Part model, mm, in its own coordinate system. Face numbers are marked on the shaded views. A direction names the side the tool comes from. Round coordinates to 2 decimals unless told otherwise and drop trailing zeros. Loops run counter-clockwise (first coordinate to the right, second up) from the corner with the lowest first, then second, coordinate; pieces in that order, holes last.
1) Band-saw the part on A-A, the plane y = 36. Write the cut outline in (x, z).
2) Band-saw the part on D-D, the plane z = -36. Write the cut outline in (x, y).
3) Drop a flat-ended pin along its axis: P1, Ø5, axis at x = -22, z = -36.5, coming from the +Y side. Give the stop position or say it passes through.
4) Band-saw the part on B-B, the plane z = 0.5. Write the cut outline in (x, y).
5) 3-axis set-ups, long thin cutter, end or side, ignore diameter. For the marked faces 1 and 2: which of +Z, -Z, +X, -X, +Y, -Y reach the whole face in a straight line?
6) Band-saw the part on C-C, the plane x = 7. Write the cut outline in (y, z).
7) Mould opens along Z. For the marked faces 3, 4, 5 and 6 say: +Z half, -Z half, draft (parallel to the pull), parting line (faces both ways), or undercut.
8) Probe line 1 (Z direction, x = 26, y = 20); line 2 (Z direction, x = -4, y = 2). List the from-to ranges inside material, lowest first.
from build123d import *

# Parameters (mm, degrees)
SKETCH1_W               = 100
SKETCH1_H               = 100
BOSS_EXTRUDE1_DEPTH     = 4
SKETCH2_W               = 100
SKETCH2_H               = 100
SKETCH2_W_2             = 92
SKETCH2_H_2             = 92
BOSS_EXTRUDE2_DEPTH     = 35
SKETCH3_W               = 4
SKETCH3_H               = 4
CUT_EXTRUDE1_DEPTH      = 4
BOSS_EXTRUDE3_DEPTH     = 2.5
SKETCH5_W               = 5.75
SKETCH5_H               = 4
CUT_EXTRUDE2_DEPTH      = 4
CUT_EXTRUDE3_DEPTH      = 79.89866919
CUT_EXTRUDE3_DEPTH_BACK = 79.89866919
SKETCH7_W               = 9.25
SKETCH7_H               = 7.5
SKETCH8_W               = 6.199178059
SKETCH8_H               = 6.70376232
SKETCH8_W_2             = 7.56876391
SKETCH8_H_2             = 7.20834658
CUT_EXTRUDE5_DEPTH      = 10
SKETCH9_W               = 12
SKETCH9_H               = 8
CUT_EXTRUDE6_DEPTH      = 10
SKETCH10_W              = 4
SKETCH10_H              = 4
BOSS_EXTRUDE4_DEPTH     = 4
SKETCH11_OUTSIDE_W      = 131.34
SKETCH11_OUTSIDE_H      = 131.34
SKETCH11_OUTSIDE_W_2    = 96
SKETCH11_OUTSIDE_H_2    = 96
CUT_EXTRUDE7_DEPTH      = 81.752708933
SKETCH12_W              = 2
SKETCH12_H              = 8
BOSS_EXTRUDE5_DEPTH     = 2


with BuildPart() as part:
    # Sketch1 → Boss-Extrude1 (new body)
    with BuildSketch(Plane(origin=(0, 0, 0), x_dir=(1, 0, 0), z_dir=(0, 1, 0))):
        Rectangle(SKETCH1_W, SKETCH1_H)
    extrude(amount=BOSS_EXTRUDE1_DEPTH)

    # Sketch2 → Boss-Extrude2 (add)
    with BuildSketch(Plane(origin=(0, 4, 0), x_dir=(1, 0, 0), z_dir=(0, 1, 0))):
        Rectangle(SKETCH2_W, SKETCH2_H)
        Rectangle(SKETCH2_W_2, SKETCH2_H_2, mode=Mode.SUBTRACT)
    extrude(amount=BOSS_EXTRUDE2_DEPTH)

    # Sketch3 → Cut-Extrude1 (cut)
    with BuildSketch(Plane(origin=(0, 0, -50), x_dir=(-1, 0, 0), z_dir=(0, 0, -1))):
        with Locations((0, 37)):
            Rectangle(SKETCH3_W, SKETCH3_H)
    extrude(amount=-CUT_EXTRUDE1_DEPTH, mode=Mode.SUBTRACT)

    # Sketch4 → Boss-Extrude3 (add)
    with BuildSketch(Plane(origin=(0, 4, 0), x_dir=(1, 0, 0), z_dir=(0, 1, 0))):
        Polygon((-1.75, -0.5), (0.75, -0.5), (0.75, 2), (-4.25, 2), (-4.25, -3), (-1.75, -3), align=None)
        Polygon((7.25, -0.5), (9.75, -0.5), (9.75, -3), (12.25, -3), (12.25, 2), (7.25, 2), align=None)
        Polygon((12.25, -14.5), (9.75, -14.5), (9.75, -17), (7.25, -17), (7.25, -19.5), (12.25, -19.5), align=None)
        Polygon((-1.75, -17), (-1.75, -14.5), (-4.25, -14.5), (-4.25, -19.5), (0.75, -19.5), (0.75, -17), align=None)
    extrude(amount=BOSS_EXTRUDE3_DEPTH)

    # Sketch5 → Cut-Extrude2 (cut)
    with BuildSketch(Plane(origin=(0, 4, 0), x_dir=(1, 0, 0), z_dir=(0, 1, 0))):
        with Locations((1.125, -15)):
            Rectangle(SKETCH5_W, SKETCH5_H)
    extrude(amount=-CUT_EXTRUDE2_DEPTH, mode=Mode.SUBTRACT)

    # Sketch7 → Cut-Extrude3 (cut, two sides: drawn at the far end of the back side and taken through both)
    with BuildSketch(Plane(origin=(0, 4, 0), x_dir=(1, 0, 0), z_dir=(0, 1, 0)).offset(-CUT_EXTRUDE3_DEPTH_BACK)):
        with Locations((0.375, -15.75)):
            Rectangle(SKETCH7_W, SKETCH7_H)
        with Locations((7.625, -1.75)):
            Rectangle(SKETCH7_W, SKETCH7_H)
    extrude(amount=CUT_EXTRUDE3_DEPTH + CUT_EXTRUDE3_DEPTH_BACK, mode=Mode.SUBTRACT)

    # Sketch8 → Cut-Extrude5 (cut)
    with BuildSketch(Plane(origin=(0, 4, 0), x_dir=(1, 0, 0), z_dir=(0, 1, 0))):
        with Locations((-1.640574957, -0.408162103)):
            Rectangle(SKETCH8_W, SKETCH8_H)
        with Locations((10.072988236, -16.951317505)):
            Rectangle(SKETCH8_W_2, SKETCH8_H_2)
    extrude(amount=CUT_EXTRUDE5_DEPTH, mode=Mode.SUBTRACT)

    # Sketch9 → Cut-Extrude6 (cut)
    with BuildSketch(Plane(origin=(0, 0, -50), x_dir=(-1, 0, 0), z_dir=(0, 0, -1))):
        with Locations((0, 19.5)):
            Rectangle(SKETCH9_W, SKETCH9_H)
    extrude(amount=-CUT_EXTRUDE6_DEPTH, mode=Mode.SUBTRACT)

    # Sketch10 → Boss-Extrude4 (add)
    with BuildSketch(Plane(origin=(0, 0, -50), x_dir=(-1, 0, 0), z_dir=(0, 0, -1))):
        with Locations((0, 37)):
            Rectangle(SKETCH10_W, SKETCH10_H)
    extrude(amount=-BOSS_EXTRUDE4_DEPTH)

    # Sketch11 outside → Cut-Extrude7 (cut, through all)
    with BuildSketch(Plane(origin=(0, 39, 0), x_dir=(1, 0, 0), z_dir=(0, 1, 0))):
        Rectangle(SKETCH11_OUTSIDE_W, SKETCH11_OUTSIDE_H)
        Rectangle(SKETCH11_OUTSIDE_W_2, SKETCH11_OUTSIDE_H_2, mode=Mode.SUBTRACT)
    extrude(amount=-CUT_EXTRUDE7_DEPTH, mode=Mode.SUBTRACT)

    # Sketch12 → Boss-Extrude5 (add)
    with BuildSketch(Plane(origin=(0, 0, -48), x_dir=(-1, 0, 0), z_dir=(0, 0, -1))):
        with Locations((-5, 19.5)):
            Rectangle(SKETCH12_W, SKETCH12_H)
        with Locations((5, 19.5)):
            Rectangle(SKETCH12_W, SKETCH12_H)
    extrude(amount=-BOSS_EXTRUDE5_DEPTH)


solid = part.part
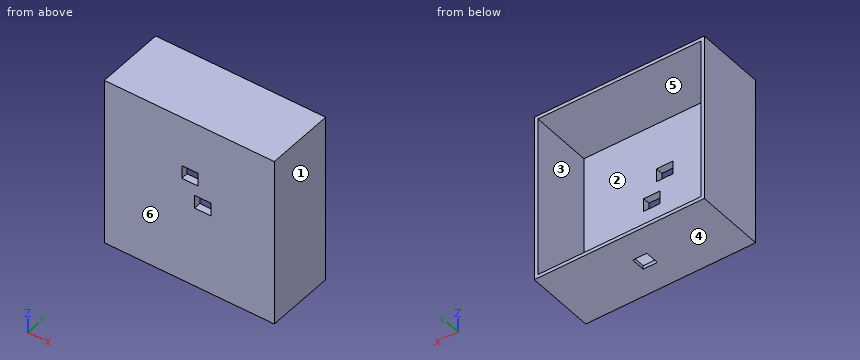
Reported:
1. outline: (-48, -48) - (48, -48) - (48, 48) - (-48, 48) - close; hole (-46, -46) - (46, -46) - (46, 46) - (-46, 46) - close
2. outline: (-48, 0) - (48, 0) - (48, 39) - (46, 39) - (46, 4) - (-46, 4) - (-46, 39) - (-48, 39) - close
3. P1: stops at y = 4
4. outline: (-48, 0) - (3, 0) - (3, 4) - (-46, 4) - (-46, 39) - (-48, 39) - close; (12.25, 0) - (48, 0) - (48, 39) - (46, 39) - (46, 4) - (12.25, 4) - close
5. face 1: +Z, -Z, +X, +Y, -Y
5. face 2: +Y
6. outline: (0, -48) - (39, -48) - (39, -46) - (4, -46) - (4, -2) - (0, -2) - close; (0, 5.5) - (4, 5.5) - (4, 46) - (39, 46) - (39, 48) - (0, 48) - close
7. face 3: undercut
7. face 4: -Z half
7. face 5: undercut
7. face 6: draft
8. line 1: z = -48 to -46, 46 to 48
8. line 2: z = -48 to 12, 19.5 to 48
